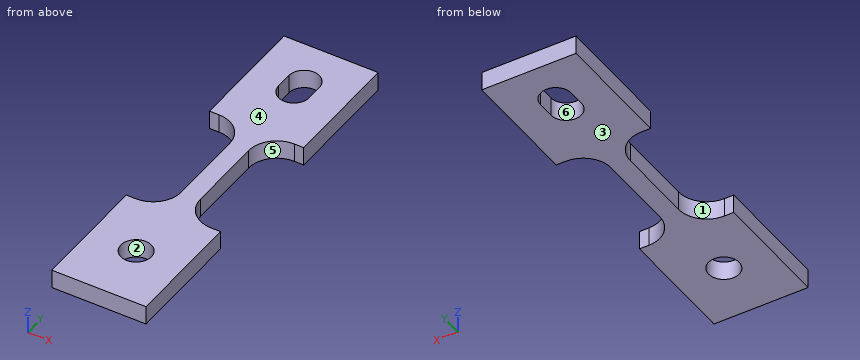
from build123d import *

# Parameters (mm, degrees)
F0_W     = 20
F0_H     = 25.5
F0_R     = 3.25
F1_DEPTH = 4
F2_W     = 4
F2_H     = 28.5
F3_DEPTH = 4
F4_R     = 6


with BuildPart() as f1:
    # F0 (on Top) → F1 (new body)
    with BuildSketch(Plane.XY):
        with Locations((0, 27)):
            Rectangle(F0_W, F0_H)
        with BuildLine():
            Line((-3.25, 27), (-3.25, 30.5))
            ThreePointArc((-3.25, 30.5), (0, 33.75), (3.25, 30.5))
            Line((3.25, 30.5), (3.25, 27))
            ThreePointArc((3.25, 27), (0, 23.75), (-3.25, 27))
        make_face(mode=Mode.SUBTRACT)
        with Locations((0, -27)):
            Rectangle(F0_W, F0_H)
        with Locations((0, -27)):
            Circle(F0_R, mode=Mode.SUBTRACT)
    extrude(amount=F1_DEPTH)

    # F2 (on Top) → F3 (join)
    with BuildSketch(Plane.XY):
        Rectangle(F2_W, F2_H)
    extrude(amount=F3_DEPTH)

    # F4
    f4_edges = [f1.edges().sort_by_distance(p)[0] for p in [
        (-2, 14.25, 2),
        (2, 14.25, 2),
        (2, -14.25, 2),
        (-2, -14.25, 2),
    ]]
    fillet(f4_edges, radius=F4_R)


solid = f1.part
Can you work these out from the model? Positions are in its coordinate system, mm. Face numbers are marked on the shaded views. A direction names the side the tool comes from. Round coordinates to 2 decimals unless told otherwise and drop trailing zeros. Write each loop counter-clockwise with the first axis right and the second up, starting at its lowest first coordinate (ties: lowest second). Pieces come first, ordered by that corner, then holes. Notation, with made-up numbers: (27, -27.5) - (48, -27.5) arc R26 ccw to (48, 2.5) - close; hole circle Ø6 at (61, 62). An arc over 180 degrees is marked (long way). Write each question's results on one line, items separated by ' | '. Start each with the question number.
1) Suppose I cut it at C-C (x = 0). List the corners of the cut face in (y, z) for me.
2) Please list where these lines run through material, in increasing order: line 1 (Y direction, x = 0, z = 2.9); line 2 (X direction, y = 28.5, z = 0.4); line 3 (Y direction, x = 8.5, z = 1.75).
3) Which directions (+Z, -Z, +X, -X, +Y, -Y) give clear straight access to the entire face, cutting with the end or side of a thin tool? Please do the marked faces 4, 5 and 6.
4) For pin 1 Ø1.2 at (y, z) = (4, 2) entering from -X, with a flat end and sliding along its axis, tell me the tip position at first contact or that it passes through.
5) Suppose I cut it at D-D (x = -5). List the corners of the cut face in (y, z) for me.
6) We'd pull the mould along X, two halves only. Please class the marked faces 1, 2 and 3: released by +X, released by -X, zero draft, split by the parting line, or undercut.
7) Suppose I cut it at A-A (y = 29.5). List the corners of the cut face in (x, z) for me.
8) Suppose I cut it at B-B (z = 2.3). List the corners of the cut face in (x, y) for me, and give its area (3 significant figures).
Here are the results:
1) outline: (-39.75, 0) - (-30.25, 0) - (-30.25, 4) - (-39.75, 4) - close; (-23.75, 0) - (23.75, 0) - (23.75, 4) - (-23.75, 4) - close; (33.75, 0) - (39.75, 0) - (39.75, 4) - (33.75, 4) - close
2) line 1: y = -39.75 to -30.25, -23.75 to 23.75, 33.75 to 39.75 | line 2: x = -10 to -3.25, 3.25 to 10 | line 3: y = -39.75 to -14.25, 14.25 to 39.75
3) face 4: +Z, +X, -X, +Y, -Y | face 5: +Z, -Z, +X | face 6: +Z, -Z
4) pin 1: stops at x = -2
5) outline: (-39.75, 0) - (-13.45, 0) - (-13.45, 4) - (-39.75, 4) - close; (13.45, 0) - (39.75, 0) - (39.75, 4) - (13.45, 4) - close
6) face 1: released by -X | face 2: undercut | face 3: zero draft
7) outline: (-10, 0) - (-3.25, 0) - (-3.25, 4) - (-10, 4) - close; (3.25, 0) - (10, 0) - (10, 4) - (3.25, 4) - close
8) outline: (-10, -39.75) - (10, -39.75) - (10, -14.25) - (8, -14.25) arc R6 cw to (2, -8.25) - (2, 8.25) arc R6 cw to (8, 14.25) - (10, 14.25) - (10, 39.75) - (-10, 39.75) - (-10, 14.25) - (-8, 14.25) arc R6 cw to (-2, 8.25) - (-2, -8.25) arc R6 cw to (-8, -14.25) - (-10, -14.25) - close; hole circle Ø6.5 at (0, -27); hole (-3.25, 27) arc R3.25 ccw to (3.25, 27) - (3.25, 30.5) arc R3.25 ccw to (-3.25, 30.5) - close | area: 1,080 mm2
